Input: part model. Units: mm. Frame: model coordinates. Give positions to 0.01 mm unless a question says otherwise; leave off trailing zeros. Loops run counter-clockwise (first coordinate to the right, second up) from the corner with the lowest first, then second, coordinate; pieces in that order, holes last.
Autodesk Inventor part; units mm, degrees
ref_plane "YZ Plane" through (0, 0, 0) normal (1, 0, 0) x (0, 1, 0)
ref_plane "XZ Plane" through (0, 0, 0) normal (0, 1, 0) x (-1, 0, 0)
ref_plane "XY Plane" through (0, 0, 0) normal (0, 0, 1) x (1, 0, 0)
sketch "Sketch1" plane through (0, 0, 0) normal (0, 0, 1) x (1, 0, 0)
  circle A0 centre (0, 0) radius 149.225
  circle A1 centre (0, 0) radius 120.2563 construction
  circle A2 centre (120.2563, 0) radius 2.5781
  circle A3 centre (0, 120.2563) radius 2.5781
  circle A4 centre (-120.2563, 0) radius 2.5781
  circle A5 centre (0, -120.2563) radius 2.5781
  line L0 (120.2563, 0) -> (0, 0) construction
  line L1 (0, 0) -> (0, 120.2563) construction
  line L2 (0, 0) -> (0, -120.2563) construction
  line L3 (0, 0) -> (-120.2563, 0) construction
  circle A6 centre (3.175, -146.05) radius 1.1557
  circle A7 centre (-3.175, -146.05) radius 1.1557
  line L4 (0, -120.2563) -> (0, -149.225) construction
  line L5 (3.175, -146.05) -> (0, -146.05) construction
  line L6 (0, -146.05) -> (-3.175, -146.05) construction
  dimension "d0" = 298.45
  dimension "d1" = 240.5126
  dimension "d2" = 5.1562
  dimension "d3" = 5.1562
  dimension "d4" = 5.1562
  dimension "d5" = 5.1562
  dimension "d8" = 2.3114
  dimension "d9" = 2.3114
  dimension "d10" = 146.05
  dimension "d11" = 3.175
extrude "Extrusion1" add sketch "Sketch1" along normal blind 3.175 contours A0 | A6 | A7
extrude "Extrusion2" cut sketch "Sketch1" along normal blind 3.175 contours A6 | A7
properties part number "roundplate" material "Aluminum 6061"
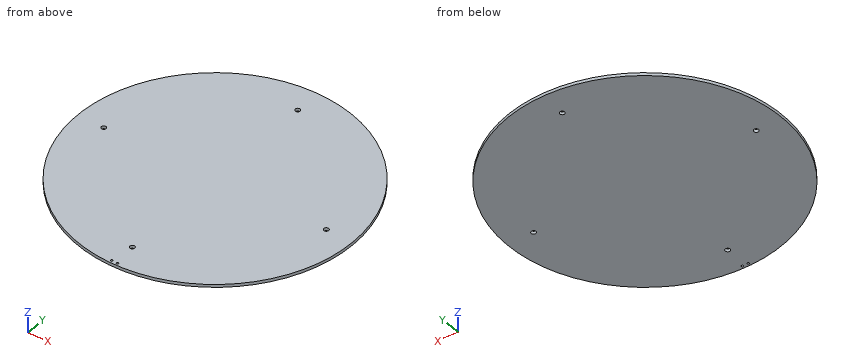
(1) Cut plane A-A (z = 0.7). Return the cut outline in (x, y) (3 decimals).
Values follow:
outline: circle Ø298.45 at (0, 0); hole circle Ø5.156 at (-120.256, 0); hole circle Ø2.311 at (-3.175, -146.05); hole circle Ø5.156 at (0, -120.256); hole circle Ø5.156 at (0, 120.256); hole circle Ø2.311 at (3.175, -146.05); hole circle Ø5.156 at (120.256, 0)
(2) Pin query (flat end, axial travel): pin 1 Ø4.5 at (x, y) = (-120.26, 0) entering from -Z; pin 2 Ø4 at (x, y) = (-2, 84.5) entering from -Z; pin 3 Ø1.5 at (y, z) = (-97.5, 2.5) entering from -X. Return the tip coordinate at first contact, or that it passes through.
Values follow:
pin 1: passes through
pin 2: stops at z = 0
pin 3: stops at x = -113.61
(3) Ray query, probe 1 along Y at (x, z) = (0, 1.9) (3 decimals); probe 2 along Y at (x, z) = (-118.5, 0.55); probe 3 along Y at (x, z) = (-24, 3). Return the intervals inside material, ascending.
Values follow:
probe 1: y = -149.225 to -122.834, -117.678 to 117.678, 122.834 to 149.225
probe 2: y = -90.7 to -1.89, 1.89 to 90.7
probe 3: y = -147.28 to 147.28
(4) Cut plane B-B (x = 67). Return the cut outline in (y, z) (3 decimals).
Values follow:
outline: (-133.338, 0) - (133.338, 0) - (133.338, 3.175) - (-133.338, 3.175) - close
(5) Cut plane C-C (y = 58). Return the cut outline in (x, z) (3 decimals).
Values follow:
outline: (-137.492, 0) - (137.492, 0) - (137.492, 3.175) - (-137.492, 3.175) - close
